Part model, mm, in its own coordinate system. A direction names the side the tool comes from. Give positions to 0.01 mm unless a question says otherwise; leave off trailing zeros. Write each loop counter-clockwise with the first axis right and the second up, starting at its lowest first coordinate (ties: lowest second). Pieces come first, ordered by that corner, then holes. Notation, with made-up numbers: M 74.5,-12.5 L 109.5,-12.5 A11 cw 109.5,-7.5 Z; hole C 86.25,-29 d9. An arc over 180 degrees is marked long. Answer as CSV lines item,"result". Start each with the question number.
Item 1: Wall check: L1, parallel to Y at x = -13.65, z = -0.3; L2, parallel to Y at x = 3, z = 1.05; L3, parallel to X at y = 4.5, z = 0.8. Give the ranges that are in metal, low to high. Write a range as from..to.
Item 2: Band-saw the part on A-A, the plane y = 4.5. List the corners of the cut face in (x, z).
Item 3: Band-saw the part on B-B, the plane x = 13.65. List the corners of the cut face in (y, z).
Item 4: Band-saw the part on C-C, the plane y = 0. List the corners of the cut face in (x, z).
Item 5: Two-plate mould, pull along Y, no slides. Class faces 4 (the cylindrical face through (12.65, 0.04, 0.02)), 5 (the flat face through (-11.5, 0, 0)), 6 (the flat face through (-18, -22, 0)), 7 (the flat face through (0, -25, 0)): +Y half, -Y half, draft (parallel to the pull), parting line (faces both ways), or undercut.
Item 6: 3-axis set-ups, long thin cutter, end or side, ignore diameter. For faces 1 (the flat face through (11.5, 0, 0)), 2 (the flat face through (0, -9, 1.5)), 3 (the flat face through (-21, -22, 0)): which of +Z, -Z, +X, -X, +Y, -Y reach the whole face in a straight line?
Item 7: Band-saw the part on D-D, the plane z = -0.4. List the corners of the cut face in (x, y).
Item 8: Pin check, flat tip, straight feed: pin 1 (0.9 mm diameter, centred on x = 19, z = 0, fed in from -Y). Stop position of the tip, or through.
from build123d import *

# Parameters (mm, degrees)
F0_W     = 50
F0_H     = 40
F1_DEPTH = 1.5
F2_W     = 23
F2_H     = 12
F2_R     = 1
F3_DEPTH = 25
F4_W     = 3
F4_H     = 6
F5_DEPTH = 25


with BuildPart() as f1:
    # F0 (on Top) → F1 (new body, symmetric)
    with BuildSketch(Plane.XY):
        with Locations((0, -5)):
            Rectangle(F0_W, F0_H)
    extrude(amount=F1_DEPTH, both=True)

    # F2 (on face) → F3 (cut)
    with BuildSketch(Plane.XY.offset(1.5)):
        Rectangle(F2_W, F2_H)
        with Locations((13.65, 0)):
            Circle(F2_R)
        with Locations((-13.65, 0)):
            Circle(F2_R)
    extrude(amount=-F3_DEPTH, mode=Mode.SUBTRACT)

    # F4 (on face) → F5 (cut)
    with BuildSketch(Plane.XY.offset(1.5)):
        with Locations((-19.5, -22)):
            Rectangle(F4_W, F4_H)
        with Locations((19.5, -22)):
            Rectangle(F4_W, F4_H)
    extrude(amount=-F5_DEPTH, mode=Mode.SUBTRACT)


solid = f1.part
Output:
1,L1,"-25..-1, 1..15"
1,L2,"-25..-6, 6..15"
1,L3,"-25..-11.5, 11.5..25"
2,outline,"M -25,-1.5 L -11.5,-1.5 L -11.5,1.5 L -25,1.5 Z; M 11.5,-1.5 L 25,-1.5 L 25,1.5 L 11.5,1.5 Z"
3,outline,"M -25,-1.5 L -1,-1.5 L -1,1.5 L -25,1.5 Z; M 1,-1.5 L 15,-1.5 L 15,1.5 L 1,1.5 Z"
4,outline,"M -25,-1.5 L -14.65,-1.5 L -14.65,1.5 L -25,1.5 Z; M -12.65,-1.5 L -11.5,-1.5 L -11.5,1.5 L -12.65,1.5 Z; M 11.5,-1.5 L 12.65,-1.5 L 12.65,1.5 L 11.5,1.5 Z; M 14.65,-1.5 L 25,-1.5 L 25,1.5 L 14.65,1.5 Z"
5,face 4,"undercut"
5,face 5,"undercut"
5,face 6,"draft"
5,face 7,"-Y half"
6,face 1,"+Z, -Z"
6,face 2,"+Z, +X, -X, +Y, -Y"
6,face 3,"+Z, -Z, -Y"
7,outline,"M -25,-25 L -21,-25 L -21,-19 L -18,-19 L -18,-25 L 18,-25 L 18,-19 L 21,-19 L 21,-25 L 25,-25 L 25,15 L -25,15 Z; hole C -13.65,0 d2; hole M -11.5,-6 L 11.5,-6 L 11.5,6 L -11.5,6 Z; hole C 13.65,0 d2"
8,pin 1,"y = -19"
